The listing builds one solid part. Answer for the finished solid, in the listing's coordinates (mm). A direction names the side the tool comes from. Coordinates: 2 decimals unless noted, no trailing zeros. Order: outer loops, then holes, each group sorted by start corner. A loop starts at its lowest first (then second) coordinate and runs counter-clockwise, first axis right, second up.
from build123d import *

# Parameters (mm, degrees)
F1_DEPTH      = 7.5
F1_DEPTH_BACK = 7.5
F2_R          = 3
F3_DEPTH      = 5.001


with BuildPart() as f1:
    # F0 (on Right) → F1 (new body, two sides)
    with BuildSketch(Plane.YZ) as f1_sk:
        with BuildLine():
            Line((-44, 1.5), (-44, 0))
            Line((-44, 0), (-33.282878, 0))
            ThreePointArc((-33.282878, 0), (-32.237053, 0.054838), (-31.202699, 0.21875))
            ThreePointArc((-31.202699, 0.21875), (-15.687375, 2.677432), (0, 3.5))
            ThreePointArc((0, 3.5), (15.687375, 2.677432), (31.202699, 0.21875))
            ThreePointArc((31.202699, 0.21875), (32.237053, 0.054838), (33.282878, 0))
            Line((33.282878, 0), (44, 0))
            Line((44, 0), (44, 1.5))
            Line((44, 1.5), (33.282878, 1.5))
            ThreePointArc((33.282878, 1.5), (32.393927, 1.546612), (31.514726, 1.685938))
            ThreePointArc((31.514726, 1.685938), (15.844249, 4.169206), (0, 5))
            ThreePointArc((0, 5), (-15.844249, 4.169206), (-31.514726, 1.685938))
            ThreePointArc((-31.514726, 1.685938), (-32.393927, 1.546612), (-33.282878, 1.5))
            Line((-33.282878, 1.5), (-44, 1.5))
        make_face()
    extrude(amount=F1_DEPTH)
    extrude(f1_sk.sketch, amount=-F1_DEPTH_BACK)

    # F2 (on Top) → F3 (cut, through all)
    with BuildSketch(Plane.XY):
        with Locations((0, 40)):
            Circle(F2_R)
        with Locations((0, -40)):
            Circle(F2_R)
    extrude(amount=F3_DEPTH, mode=Mode.SUBTRACT)


solid = f1.part
1) Section D-D (y = -27) is taken. Give the vertices of the cut face in (x, z).
2) Section C-C (x = -3.75) is taken. Give the vertices of the cut face in (y, z), then the cut area to 3 significant figures.
3) Section A-A (x = 0) is taken. Give the vertices of the cut face in (y, z), then the cut area to 3 significant figures.
4) Determine the mould class of faces 1 (the face through (0, 44, 1)), 2 (the face through (0, 43, 1)), 3 (the face through (-7.5, 0, 4)) for opening direction X: released by +X, released by -X, zero draft, split by the parting line, or undercut.
5) Consider L1, parallel to X at y = -40, z = 0.7; L2, parallel to Z at x = -4.5, y = -1; L3, parallel to Z at x = 4.5, y = 6. Determine where each line is inside the solid, lowest interval first.
6) Each of these flat-tipped pins is pushed along its axis until it touches: P1, Ø1.5, axis at x = -1.5, y = -21, coming from the +Z side; P2, Ø7, axis at x = 0, y = 40, coming from the +Z side; P3, Ø8, axis at x = 2, y = 23, coming from the +Z side. Where does it stop, or does it pass through?
7) A tool of negligible diameter and unlimited length cuts with its end or side. For faces 4 (the face through (0, 36, 1.5)), 5 (the face through (2, -37, 1.5)), 6 (the face through (7.5, 0, 4)), 7 (the face through (0.105, 32.222, 0.056)), 8 (the face through (0, -37, 1)), from which of +Z, -Z, +X, -X, +Y, -Y can it reach the whole face along a straight path? Write none if from no direction.
8) Section B-B (y = 40) is taken. Give the vertices of the cut face in (x, z), then the cut area to 3 significant figures.
Filled sheet:
1. outline: (-7.5, 1.05) - (7.5, 1.05) - (7.5, 2.57) - (-7.5, 2.57) - close
2. outline: (-44, 0) - (-33.28, 0) arc R10 ccw to (-31.2, 0.22) arc R150 cw to (0, 3.5) arc R150 cw to (31.2, 0.22) arc R10 ccw to (33.28, 0) - (44, 0) - (44, 1.5) - (33.28, 1.5) arc R8.5 cw to (31.51, 1.69) arc R151.5 ccw to (0, 5) arc R151.5 ccw to (-31.51, 1.69) arc R8.5 cw to (-33.28, 1.5) - (-44, 1.5) - close
2. area: 133 mm2
3. outline: (-44, 0) - (-43, 0) - (-43, 1.5) - (-44, 1.5) - close; (-37, 0) - (-33.28, 0) arc R10 ccw to (-31.2, 0.22) arc R150 cw to (0, 3.5) arc R150 cw to (31.2, 0.22) arc R10 ccw to (33.28, 0) - (37, 0) - (37, 1.5) - (33.28, 1.5) arc R8.5 cw to (31.51, 1.69) arc R151.5 ccw to (0, 5) arc R151.5 ccw to (-31.51, 1.69) arc R8.5 cw to (-33.28, 1.5) - (-37, 1.5) - close; (43, 0) - (44, 0) - (44, 1.5) - (43, 1.5) - close
3. area: 115 mm2
4. face 1: zero draft
4. face 2: undercut
4. face 3: released by -X
5. L1: x = -7.5 to -3, 3 to 7.5
5. L2: z = 3.5 to 5
5. L3: z = 3.38 to 4.88
6. P1: stops at z = 3.64
6. P2: stops at z = 1.5
6. P3: stops at z = 3.8
7. face 4: +Z, +X, -X, +Y
7. face 5: +Z, +X, -X, -Y
7. face 6: +Z, -Z, +X, +Y, -Y
7. face 7: -Z, +X, -X
7. face 8: +Z, -Z
8. outline: (-7.5, 0) - (-3, 0) - (-3, 1.5) - (-7.5, 1.5) - close; (3, 0) - (7.5, 0) - (7.5, 1.5) - (3, 1.5) - close
8. area: 13.5 mm2
